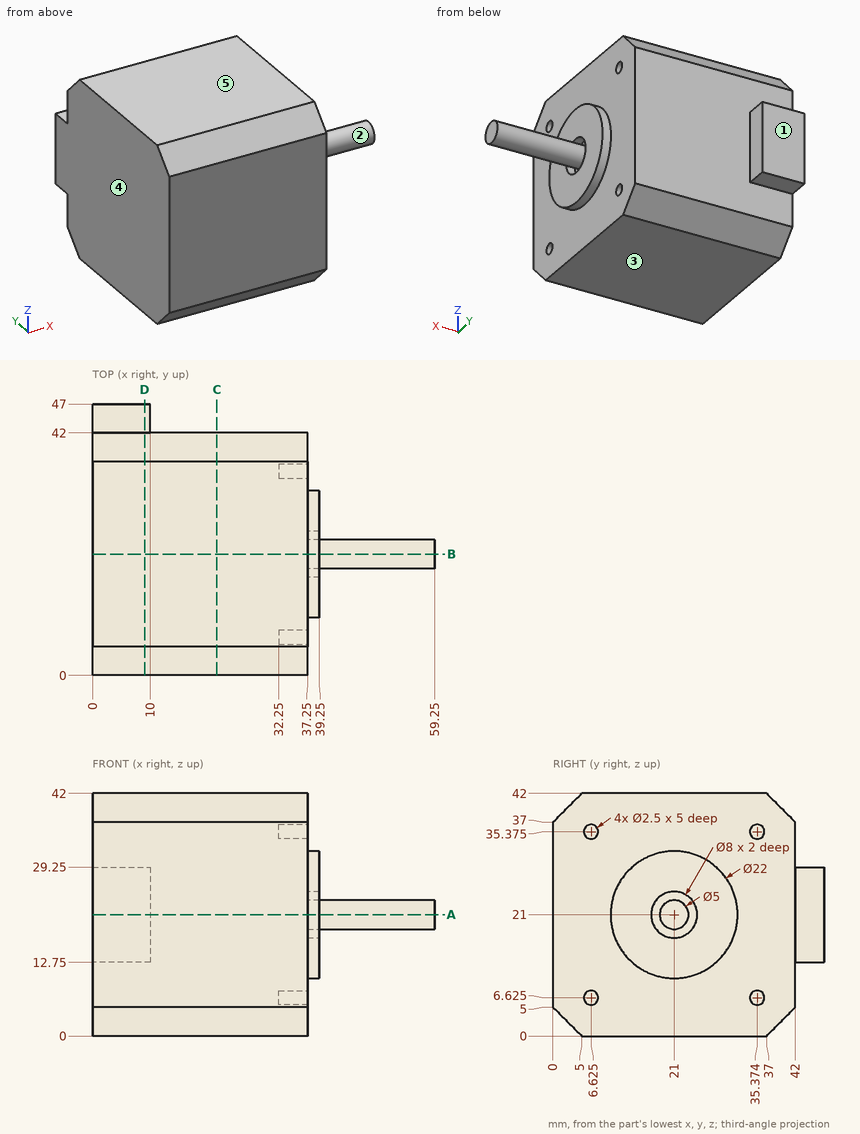
Answer from the drawing. Dimensions are ordinates in mm from the lowest x, y and z of the part. A direction names the side the tool comes from. Give positions to 0.01 mm unless a question says otherwise; leave off trailing zeros. Loops run counter-clockwise (first coordinate to the right, second up) from the corner with the lowest first, then second, coordinate; pieces in that order, holes last.
Item 1: A cutting plane is placed at C-C (x = 21.5). Give the vertices of the cut face in (y, z).
Derived:
outline: (0, 5) - (5, 0) - (37, 0) - (42, 5) - (42, 37) - (37, 42) - (5, 42) - (0, 37) - close
Item 2: Determine the mould class of the marked faces 3, 4 and 5 for opening direction Z: +Z half, -Z half, draft (parallel to the pull), parting line (faces both ways), or undercut.
Derived:
face 3: -Z half
face 4: draft
face 5: +Z half
Item 3: Each of these flat-tipped pins is pushed along its axis until it touches: pin 1 Ø6 at (y, z) = (8.5, 14.5) entering from +X; pin 2 Ø5.5 at (x, y) = (7, 45) entering from +Z; pin 3 Ø0.8 at (y, z) = (35, 6.5) entering from +X. Where does it stop, or does it pass through?
Derived:
pin 1: stops at x = 37.25
pin 2: stops at z = 29.25
pin 3: stops at x = 32.25
Item 4: A cutting plane is placed at A-A (z = 21). Give the vertices of the cut face in (x, y), then the cut area to 3 significant figures.
Derived:
outline: (0, 0) - (37.25, 0) - (37.25, 10) - (39.25, 10) - (39.25, 17) - (37.25, 17) - (37.25, 18.5) - (59.25, 18.5) - (59.25, 23.5) - (37.25, 23.5) - (37.25, 25) - (39.25, 25) - (39.25, 32) - (37.25, 32) - (37.25, 42) - (10, 42) - (10, 47) - (0, 47) - close
area: 1,750 mm2
Item 5: A cutting plane is placed at D-D (x = 9). Give the vertices of the cut face in (y, z), then the cut area to 3 significant figures.
Derived:
outline: (0, 5) - (5, 0) - (37, 0) - (42, 5) - (42, 12.75) - (47, 12.75) - (47, 29.25) - (42, 29.25) - (42, 37) - (37, 42) - (5, 42) - (0, 37) - close
area: 1,800 mm2
Item 6: Find the intervals of material crossed by line 1 along X through (y, z) = (13, 21); line 2 along Y through (x, z) = (31, 20); line 3 along X through (y, z) = (11.5, 34), in increasing order.
Derived:
line 1: x = 0 to 39.25
line 2: y = 0 to 42
line 3: x = 0 to 37.25
Item 7: A tool of negligible diameter and unlimited length cuts with its end or side. For the marked faces 1 and 2, from which of +Z, -Z, +X, -X, +Y, -Y can it reach the whole face along a straight path? Write none if from no direction.
Derived:
face 1: +Z, -Z, +X, -X, +Y
face 2: +X
Item 8: A cutting plane is placed at B-B (y = 21). Give the vertices of the cut face in (x, z), then the cut area to 3 significant figures.
Derived:
outline: (0, 0) - (37.25, 0) - (37.25, 10) - (39.25, 10) - (39.25, 17) - (37.25, 17) - (37.25, 18.5) - (59.25, 18.5) - (59.25, 23.5) - (37.25, 23.5) - (37.25, 25) - (39.25, 25) - (39.25, 32) - (37.25, 32) - (37.25, 42) - (0, 42) - close
area: 1,700 mm2
